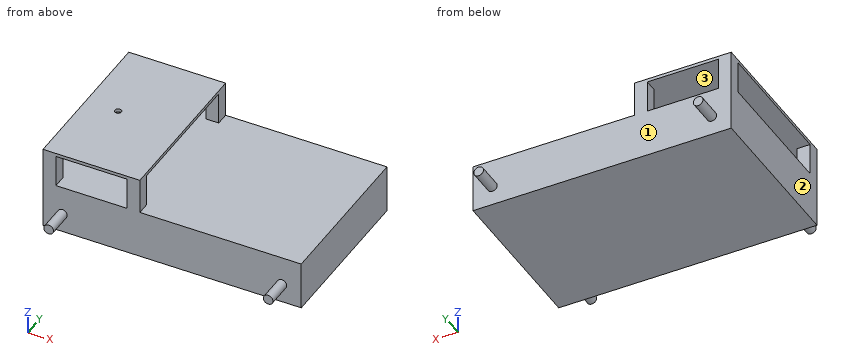
```python
from build123d import *

# Parameters (mm, degrees)
SKETCH1_W           = 400
SKETCH1_H           = 250
BOSS_EXTRUDE1_DEPTH = 5
SKETCH2_W           = 20
SKETCH2_H           = 20
SKETCH2_W_2         = 16
SKETCH2_H_2         = 16
BOSS_EXTRUDE3_DEPTH = 50
SKETCH3_W           = 150
SKETCH3_H           = 250
BOSS_EXTRUDE4_DEPTH = 5
SKETCH4_R           = 5
CUT_EXTRUDE1_DEPTH  = 5
SKETCH5_W           = 400
SKETCH5_H           = 250
SKETCH5_W_2         = 390
SKETCH5_H_2         = 240
BOSS_EXTRUDE5_DEPTH = 70
SKETCH6_W           = 400
SKETCH6_H           = 250
BOSS_EXTRUDE6_DEPTH = 5
SKETCH7_R           = 7.5
BOSS_EXTRUDE7_DEPTH = 40
BOSS_EXTRUDE8_START = 40
SKETCH8_R           = 7.5
BOSS_EXTRUDE8_DEPTH = 40


with BuildPart() as part:
    # Sketch1 → Boss-Extrude1 (new body)
    with BuildSketch(Plane.XY):
        with Locations((200, -125)):
            Rectangle(SKETCH1_W, SKETCH1_H)
    extrude(amount=BOSS_EXTRUDE1_DEPTH)

    # Sketch2 → Boss-Extrude3 (add)
    # profile 1 of 4: a face of its own
    with BuildSketch(Plane.XY.offset(5)):
        with Locations((10, -240)):
            Rectangle(SKETCH2_W, SKETCH2_H)
        with Locations((10, -240)):
            Rectangle(SKETCH2_W_2, SKETCH2_H_2, mode=Mode.SUBTRACT)
    # profile 2 of 4: a face of its own
    with BuildSketch(Plane.XY.offset(5)):
        with Locations((140, -240)):
            Rectangle(SKETCH2_W, SKETCH2_H)
        with Locations((140, -240)):
            Rectangle(SKETCH2_W_2, SKETCH2_H_2, mode=Mode.SUBTRACT)
    # profile 3 of 4: a face of its own
    with BuildSketch(Plane.XY.offset(5)):
        with Locations((10, -10)):
            Rectangle(SKETCH2_W, SKETCH2_H)
        with Locations((10, -10)):
            Rectangle(SKETCH2_W_2, SKETCH2_H_2, mode=Mode.SUBTRACT)
    # profile 4 of 4: a face of its own
    with BuildSketch(Plane.XY.offset(5)):
        with Locations((140, -10)):
            Rectangle(SKETCH2_W, SKETCH2_H)
        with Locations((140, -10)):
            Rectangle(SKETCH2_W_2, SKETCH2_H_2, mode=Mode.SUBTRACT)
    extrude(amount=BOSS_EXTRUDE3_DEPTH)

    # Sketch3 → Boss-Extrude4 (add)
    with BuildSketch(Plane.XY.offset(55)):
        with Locations((75, -125)):
            Rectangle(SKETCH3_W, SKETCH3_H)
    extrude(amount=BOSS_EXTRUDE4_DEPTH)

    # Sketch4 → Cut-Extrude1 (cut)
    with BuildSketch(Plane.XY.offset(60)):
        with Locations((50, -125)):
            Circle(SKETCH4_R)
    extrude(amount=-CUT_EXTRUDE1_DEPTH, mode=Mode.SUBTRACT)

    # Sketch5 → Boss-Extrude5 (add)
    with BuildSketch(Plane(origin=(0, 0, 0), x_dir=(-1, 0, 0), z_dir=(0, 0, -1))):
        with Locations((-200, -125)):
            Rectangle(SKETCH5_W, SKETCH5_H)
        with Locations((-200, -125)):
            Rectangle(SKETCH5_W_2, SKETCH5_H_2, mode=Mode.SUBTRACT)
    extrude(amount=BOSS_EXTRUDE5_DEPTH)

    # Sketch6 → Boss-Extrude6 (add)
    with BuildSketch(Plane(origin=(0, 0, -70), x_dir=(-1, 0, 0), z_dir=(0, 0, -1))):
        with Locations((-200, -125)):
            Rectangle(SKETCH6_W, SKETCH6_H)
    extrude(amount=-BOSS_EXTRUDE6_DEPTH)

    # Sketch7 → Boss-Extrude7 (add)
    with BuildSketch(Plane.XZ.offset(250)):
        with Locations(Location((30, -40, 0), (0, 0, 90))):
            Circle(SKETCH7_R)
        with Locations(Location((370, -40, 0), (0, 0, 90))):
            Circle(SKETCH7_R)
    extrude(amount=BOSS_EXTRUDE7_DEPTH)

    # Sketch8 → Boss-Extrude8 (add)
    with BuildSketch(Plane(origin=(0, 0, 0), x_dir=(1, 0, 0), z_dir=(0, 1, 0)).offset(BOSS_EXTRUDE8_START)):
        with Locations(Location((370, 40, 0), (0, 0, 270))):
            Circle(SKETCH8_R)
        with Locations(Location((30, 40, 0), (0, 0, 270))):
            Circle(SKETCH8_R)
    extrude(amount=-BOSS_EXTRUDE8_DEPTH)


solid = part.part
```
Work out the finished part from the listing and answer in its coordinate system (mm). Face numbers are marked on the shaded views. Give positions to 0.01 mm unless a question says otherwise; leave off trailing zeros. Write each loop counter-clockwise with the first axis right and the second up, starting at its lowest first coordinate (ties: lowest second). Pieces come first, ordered by that corner, then holes. Notation, with made-up numbers: (52.25, -38) -> (69.25, -38) arc R28 ccw to (69.25, -7) -> close; hole circle Ø6 at (5.5, 28). An arc over 180 degrees is marked (long way). Write item = value, one per line.
Q1. For a pull along Y with two mould halves and no side action, classify the marked faces 1, 2 and 3 as pulls with the +Y half, pulls with the -Y half, needs draft (parallel to the pull), parting line crosses it, or undercut.
Computed values:
face_1 = pulls with the +Y half
face_2 = needs draft
face_3 = undercut
Q2. Consider line 1 along Z through (x, y) = (127.5, -25); line 2 along Y through (x, z) = (50, 57); line 3 along Z through (x, y) = (212.5, -184.5). Determine where each line is inside the solid, lowest interval first.
Computed values:
line_1 = -70 to -65, 0 to 5, 55 to 60
line_2 = -250 to -130, -120 to 0
line_3 = -70 to -65, 0 to 5
Q3. Flat-ended cylindrical pins translate along their axes: pin 1 Ø3 at (x, y) = (212, -130.5) entering from +Z; pin 2 Ø17.5 at (y, z) = (-8.5, 18) entering from +X; pin 3 Ø19.5 at (x, z) = (179.5, -41.5) entering from -Y. Find the tip coordinate at first contact, or state that the pin passes through.
Computed values:
pin_1 = 5
pin_2 = 150
pin_3 = -250
Q4. Section B-B on x = 113 is taken. Determine the outline of the cut face in (y, z).
Computed values:
outline = (-250, -70) -> (0, -70) -> (0, 5) -> (-250, 5) -> close; (-250, 55) -> (0, 55) -> (0, 60) -> (-250, 60) -> close; hole (-245, -65) -> (-5, -65) -> (-5, 0) -> (-245, 0) -> close
Q5. Section A-A on y = -125 is taken. Determine the outline of the cut face in (x, z).
Computed values:
outline = (0, -70) -> (400, -70) -> (400, 5) -> (0, 5) -> close; (0, 55) -> (45, 55) -> (45, 60) -> (0, 60) -> close; (55, 55) -> (150, 55) -> (150, 60) -> (55, 60) -> close; hole (5, -65) -> (395, -65) -> (395, 0) -> (5, 0) -> close
Q6. Section C-C on z = 18 is taken. State how many separate pieces and enclosed holes the cut face has, and give its area (3 significant figures).
Computed values:
separate_pieces = 4
enclosed_holes = 4
area = 576 mm^2
Q7. Section D-D on x = 50 is taken. Determine the outline of the cut face in (y, z), and give its area (3 significant figures).
Computed values:
outline = (-250, -70) -> (0, -70) -> (0, 5) -> (-250, 5) -> close; (-250, 55) -> (-130, 55) -> (-130, 60) -> (-250, 60) -> close; (-120, 55) -> (0, 55) -> (0, 60) -> (-120, 60) -> close; hole (-245, -65) -> (-5, -65) -> (-5, 0) -> (-245, 0) -> close
area = 4,350 mm^2
